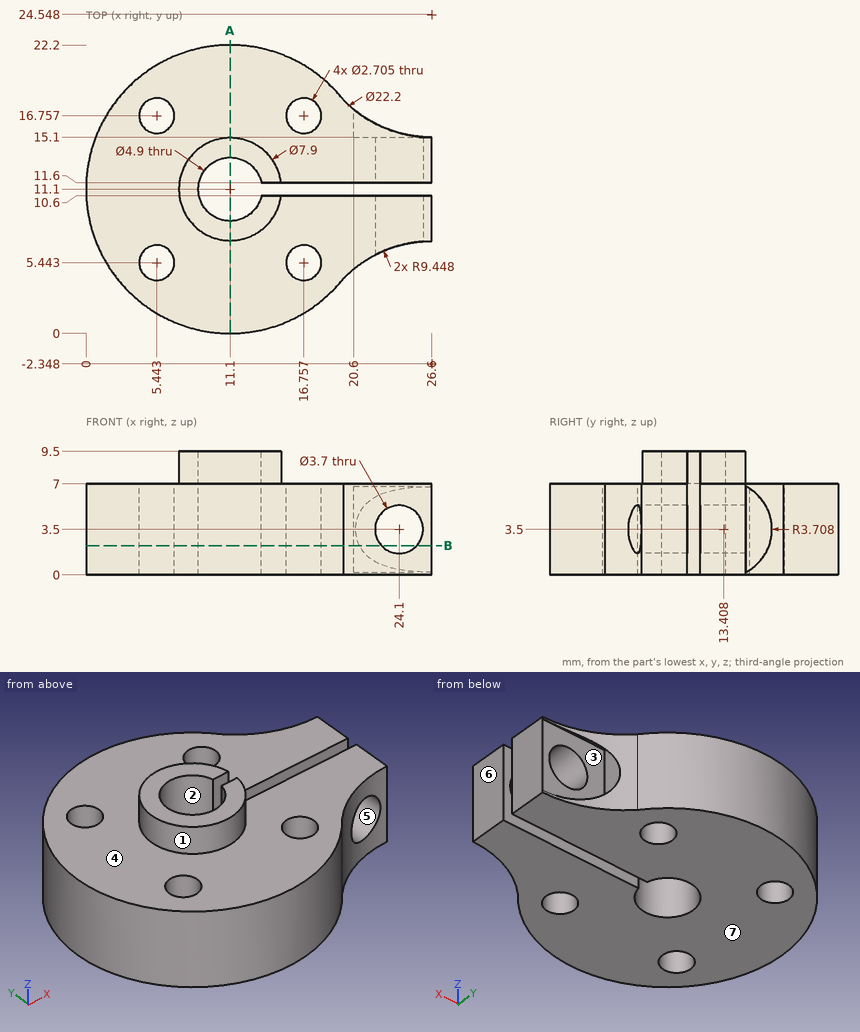
Geometry check sheet. Reference: drawing and pictorial views, mm from the part's lowest x, y, z. A direction names the side the tool comes from. Give positions to 0.01 mm unless a question says otherwise; leave off trailing zeros. Order: outer loops, then holes, each group sorted by start corner. A loop starts at its lowest first (then second) coordinate and runs counter-clockwise, first axis right, second up.
1. Access from +Z, -Z, +X, -X, +Y, -Y to the whole of each face (thin tool, end or side, straight path). Record for the marked faces 1, 2 and 3.
2. Section check B-B, the plane z = 2.25. Give the number of separate pieces and of enclosed holes in the cut face, and give its area (3 significant figures).
3. Section check A-A, the plane x = 11.1. Enter the section's corners in (y, z).
4. Release check for a two-part mould opening along Z. For the marked faces 4, 5, 6 and 7 record: pulls with the +Z half, pulls with the -Z half, needs draft (parallel to the pull), parting line crosses it, or undercut.
5. Thickness scan on L1, parallel to X at y = 9.25, z = 2.5 (1 decimal); L2, parallel to X at y = 10.5, z = 4 (1 decimal); L3, parallel to Z at x = 8, y = 15.5. Record the ranges inside material, lowest first.
6. Gauge pin test, flat ends, axial feed: pin 1 Ø8 at (x, y) = (21, 11.5) entering from +Z; pin 2 Ø0.6 at (y, z) = (16.5, 2.5) entering from +X; pin 3 Ø4 at (x, z) = (13.5, 8.5) entering from -Y. Record the tip position at first contact, or that the pin passes through.
Values follow:
1. face 1: +Z
1. face 2: +Z, -Z
1. face 3: +X
2. separate pieces: 3
2. enclosed holes: 4
2. area: 352 mm2
3. outline: (0, 0) - (8.65, 0) - (8.65, 9.5) - (7.15, 9.5) - (7.15, 7) - (0, 7) - close; (13.55, 0) - (22.2, 0) - (22.2, 7) - (15.05, 7) - (15.05, 9.5) - (13.55, 9.5) - close
4. face 4: pulls with the +Z half
4. face 5: undercut
4. face 6: needs draft
4. face 7: pulls with the -Z half
5. L1: x = 0.2 to 9.5, 12.7 to 22.5, 25.7 to 26.6
5. L2: x = 0 to 8.7, 13.5 to 22.3, 25.9 to 26.6
5. L3: z = 0 to 7
6. pin 1: stops at z = 7
6. pin 2: stops at x = 20.6
6. pin 3: stops at y = 0.05
